```python
from build123d import *

# Parameters (mm, degrees)
SKETCH1_W           = 65
SKETCH1_H           = 25
BOSS_EXTRUDE1_DEPTH = 3
BOSS_EXTRUDE2_DEPTH = 17
SKETCH2_3_W         = 2
SKETCH2_3_H         = 21
BOSS_EXTRUDE3_DEPTH = 9


with BuildPart() as part:
    # Sketch1 → Boss-Extrude1 (new body)
    with BuildSketch(Plane(origin=(0, 0, 0), x_dir=(1, 0, 0), z_dir=(0, 1, 0))):
        with Locations((32.5, -12.5)):
            Rectangle(SKETCH1_W, SKETCH1_H)
    extrude(amount=BOSS_EXTRUDE1_DEPTH)

    # Sketch2 → Boss-Extrude2 (add)
    with BuildSketch(Plane(origin=(0, 3, 0), x_dir=(1, 0, 0), z_dir=(0, 1, 0))):
        Polygon((63, -23), (2, -23), (0, -23), (0, -25), (65, -25), (65, -23), align=None)
        Polygon((0, -2), (2, -2), (63, -2), (65, -2), (65, 0), (0, 0), align=None)
    extrude(amount=BOSS_EXTRUDE2_DEPTH)

    # Sketch2_3 → Boss-Extrude3 (add)
    with BuildSketch(Plane(origin=(0, 3, 0), x_dir=(1, 0, 0), z_dir=(0, 1, 0))):
        with Locations((1, -12.5)):
            Rectangle(SKETCH2_3_W, SKETCH2_3_H)
        with Locations((64, -12.5)):
            Rectangle(SKETCH2_3_W, SKETCH2_3_H)
    extrude(amount=BOSS_EXTRUDE3_DEPTH)


solid = part.part
```
The listing builds one solid part. Answer for the finished solid, in the listing's coordinates (mm). A direction names the side the tool comes from. Round coordinates to 2 decimals unless told otherwise and drop trailing zeros. Loops run counter-clockwise (first coordinate to the right, second up) from the corner with the lowest first, then second, coordinate; pieces in that order, holes last. Notation, with made-up numbers: (-36, -2.75) - (-29, -2.75) arc R28 cw to (-29, 31.25) - close; hole circle Ø9 at (-12, 33). An arc over 180 degrees is marked (long way). Return JSON: item names as keys, results as strings. Group by question number.
1. The part is cut by section B-B on x = 13.5. Determine the outline of the cut face in (y, z).
2. Each of these flat-tipped pins is pushed along its axis until it touches: P1, Ø1.5, axis at y = 8, z = 18, coming from the -X side; P2, Ø1.6, axis at x = 1.5, z = 12, coming from the +Y side. Where does it stop, or does it pass through?
3. The part is cut by section D-D on z = 7.75. Determine the outline of the cut face in (x, y), then the cut area to 3 significant figures.
4. The mould has two halves that part along X. Classify faces 1 (the flat face through (32, 10, 25)), 2 (the flat face through (32, 3, 12)), 3 (the flat face through (65, 8, 13)): pulls with the +X half, pulls with the -X half, needs draft (parallel to the pull), parting line crosses it, or undercut.
5. Which of the six approach directions +Z, -Z, +X, -X, +Y, -Y give full straight-line access (tool end or side, diameter ignored) to faces 4 (the flat face through (0, 8, 13)), 5 (the flat face through (2, 7, 13)), 6 (the flat face through (64, 12, 12))?
6. Consider probe 1 along X at (y, z) = (8, 3.25); probe 2 along Z at (x, y) = (19.5, 14.25); probe 3 along Y at (x, z) = (16.5, 7). Determine where each line is inside the solid, lowest interval first.
7. The part is cut by section A-A on y = 15. Determine the outline of the cut face in (x, z).
8. The part is cut by section C-C on y = 9. Determine the outline of the cut face in (x, z), then the cut area to 3 significant figures.
Resolved:
{
 "1": {"outline": "(0, 0) - (20, 0) - (20, 2) - (3, 2) - (3, 23) - (20, 23) - (20, 25) - (0, 25) - close"},
 "2": {"P1": "stops at x = 0", "P2": "stops at y = 12"},
 "3": {"outline": "(0, 0) - (65, 0) - (65, 12) - (63, 12) - (63, 3) - (2, 3) - (2, 12) - (0, 12) - close", "area": "231 mm²"},
 "4": {"face 1": "needs draft", "face 2": "undercut", "face 3": "pulls with the +X half"},
 "5": {"face 4": "+Z, -Z, -X, +Y, -Y", "face 5": "+Y", "face 6": "+X, -X, +Y"},
 "6": {"probe 1": "x = 0 to 2, 63 to 65", "probe 2": "z = 0 to 2, 23 to 25", "probe 3": "y = 0 to 3"},
 "7": {"outline": "(0, 0) - (65, 0) - (65, 2) - (0, 2) - close; (0, 23) - (65, 23) - (65, 25) - (0, 25) - close"},
 "8": {"outline": "(0, 0) - (65, 0) - (65, 25) - (0, 25) - close; hole (2, 2) - (63, 2) - (63, 23) - (2, 23) - close", "area": "344 mm²"}
}
